Part model, mm, in its own coordinate system. Round coordinates to 2 decimals unless told otherwise and drop trailing zeros. Write each loop counter-clockwise with the first axis right and the second up, starting at its lowest first coordinate (ties: lowest second). Pieces come first, ordered by that corner, then holes. Notation, with made-up numbers: (-32, 52.5) -> (-1, 52.5) arc R11 ccw to (-1, 61.5) -> close; hole circle Ø10 at (65.5, 22.25). An arc over 180 degrees is marked (long way). Return JSON: item names as keys, results as strings. Group by question number.
(1) Saw through at B-B (z = 2.4). State how many separate pieces and enclosed holes the cut face has, plus the area to 3 significant figures.
(2) Mould opens along X. For faces 1 (the cylindrical face through (-45.007, -8.894, 2.535)), 2 (the cylindrical face through (-11.923, -53.692, 2.465)), 3 (the flat face through (-1, 1, 5)), 4 (the cylindrical face through (-36.675, 26.891, 2.535)) say: +X half, -X half, draft (parallel to the pull), parting line (faces both ways), or undercut.
(3) Saw through at C-C (y = 45). List the corners of the cut face in (x, z), plus the area to 3 significant figures.
(4) Drop flat-ended pins along their axis: pin 1 Ø3 at (x, y) = (42.65, -9.74) entering from +Z; pin 2 Ø1 at (y, z) = (36, 3.5) entering from -X; pin 3 Ø3 at (x, z) = (-1, 3.5) entering from -Y. Give the stop position or say it passes through.
(5) Saw through at A-A (x = 0). List the corners of the cut face in (y, z), plus the area to 3 significant figures.
(6) Drill centre lines: L1, parallel to Y at x = 33, z = 1.1; L2, parallel to X at y = -11, z = 0.7; L3, parallel to X at y = 27, z = 4.15. Where is each one in solid material? Low to high. Write a range as from..to.
(7) Saw through at D-D (y = -43.75). List the corners of the cut face in (x, z), plus the area to 3 significant figures.
from build123d import *

# Parameters (mm, degrees)
F0_R            = 55
F1_DEPTH        = 5
F2_R            = 2.5
F3_DEPTH        = 5.001
F3_COPIES_COUNT = 14


# Not quite as in the source:
# - a pattern or mirror of a feature is missing from the dataset's text; its kind, count and spacing are read off the source's solid


with BuildPart() as f1:
    # F0 (on Top) → F1 (new body)
    with BuildSketch(Plane.XY):
        Circle(F0_R)
    extrude(amount=F1_DEPTH)

    # F2 (on face) → F3 (cut, through all)
    with BuildSketch(Plane.XY.offset(5)):
        with Locations((0, 43.75)):
            Circle(F2_R)
    f3 = extrude(amount=-F3_DEPTH, mode=Mode.SUBTRACT)

    # F3_copies: F3 ×14 about axis
    f3_copies_axis = Axis((0, 0, 0), (0, 0, 1))
    for i in range(1, F3_COPIES_COUNT):
        add(f3.rotate(f3_copies_axis, i * 360 / F3_COPIES_COUNT), mode=Mode.SUBTRACT)


solid = f1.part
Computed values:
{
 "1": {"separate pieces": "1", "enclosed holes": "14", "area": "9,230 mm2"},
 "2": {"face 1": "undercut", "face 2": "parting line", "face 3": "draft", "face 4": "undercut"},
 "3": {"outline": "(-31.62, 0) -> (-2.17, 0) -> (-2.17, 5) -> (-31.62, 5) -> close; (2.17, 0) -> (31.62, 0) -> (31.62, 5) -> (2.17, 5) -> close", "area": "295 mm2"},
 "4": {"pin 1": "through", "pin 2": "x = -42.01", "pin 3": "y = -55"},
 "5": {"outline": "(-55, 0) -> (-46.25, 0) -> (-46.25, 5) -> (-55, 5) -> close; (-41.25, 0) -> (41.25, 0) -> (41.25, 5) -> (-41.25, 5) -> close; (46.25, 0) -> (55, 0) -> (55, 5) -> (46.25, 5) -> close", "area": "500 mm2"},
 "6": {"L1": "-44..-29.47, -25.09..25.09, 29.47..44", "L2": "-53.89..-44.81, -40.5..40.5, 44.81..53.89", "L3": "-47.92..-36.69, -31.72..31.72, 36.69..47.92"},
 "7": {"outline": "(-33.33, 0) -> (-2.5, 0) -> (-2.5, 5) -> (-33.33, 5) -> close; (2.5, 0) -> (33.33, 0) -> (33.33, 5) -> (2.5, 5) -> close", "area": "308 mm2"}
}
